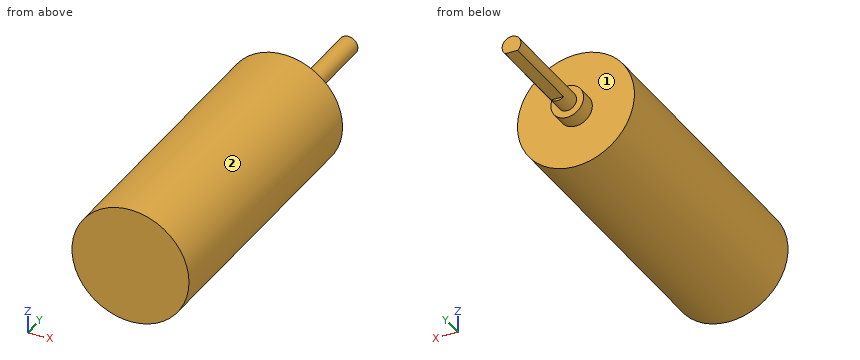
from build123d import *

# Parameters (mm, degrees)
SKETCH_1_R          = 12.5
EXTRUDE_1_DEPTH     = 62
SKETCH_2_R          = 3.5
EXTRUDE_2_DEPTH     = 3.5
SKETCH_3_R          = 2
EXTRUDE_3_DEPTH     = 22.5
CUT_EXTRUDE_1_DEPTH = 18.5


with BuildPart() as part:
    # 草图1 → 凸台-拉伸1 (new body)
    with BuildSketch(Plane(origin=(0, 0, 0), x_dir=(1, 0, 0), z_dir=(0, 1, 0))):
        Circle(SKETCH_1_R)
    extrude(amount=EXTRUDE_1_DEPTH)

    # 草图2 → 凸台-拉伸2 (add)
    with BuildSketch(Plane(origin=(0, 62, 0), x_dir=(1, 0, 0), z_dir=(0, 1, 0))):
        Circle(SKETCH_2_R)
    extrude(amount=EXTRUDE_2_DEPTH)

    # 草图3 → 凸台-拉伸3 (add)
    with BuildSketch(Plane(origin=(0, 65.5, 0), x_dir=(1, 0, 0), z_dir=(0, 1, 0))):
        Circle(SKETCH_3_R)
    extrude(amount=EXTRUDE_3_DEPTH)

    # 草图4 → 切除-拉伸1 (cut)
    with BuildSketch(Plane(origin=(0, 88, 0), x_dir=(1, 0, 0), z_dir=(0, 1, 0))):
        Polygon((-50.671161076, 1.5), (-1.322875656, 1.5), (1.322875656, 1.5), (50.671161076, 1.5), (50.671161076, 100.196570842), (-50.671161076, 100.196570842), align=None)
    extrude(amount=-CUT_EXTRUDE_1_DEPTH, mode=Mode.SUBTRACT)


solid = part.part
Input: part model. Units: mm. Frame: model coordinates. Face numbers are marked on the shaded views. A direction names the side the tool comes from. Give positions to 0.01 mm unless a question says otherwise; leave off trailing zeros. Loops run counter-clockwise (first coordinate to the right, second up) from the corner with the lowest first, then second, coordinate; pieces in that order, holes last. Notation, with made-up numbers: M 43,20.25 L 88,20.25 A18 ccw 88,47.25 Z; hole C 68,21.25 d8. An arc over 180 degrees is marked long. Use CSV: the item, a comma, the result in double quotes.
(1) Pin query (flat end, axial travel): P1, Ø4, axis at y = 77.5, z = -4.5, coming from the -X side; P2, Ø10, axis at x = -3.5, z = 5, coming from the +Y side; P3, Ø6, axis at y = 31.5, z = 6.5, coming from the +X side; P4, Ø3, axis at x = 0, y = 76, coming from the -Z side. Return the tip coordinate at first contact, or that it passes through.
Outcome:
P1,"passes through"
P2,"stops at y = 88"
P3,"stops at x = 12"
P4,"stops at z = -1.5"
(2) Set-up query: the marked faces 1 and 2. Return all of +Z, -Z, +X, -X, +Y, -Y with unobstructed straight access to the full face (end or side cutting, diameter ignored); none if empty.
Outcome:
face 1,"+Y"
face 2,"+Y, -Y"
(3) Section D-D, the plane y = 45.5. Return loops of the section in (x, z), plus the area to 3 significant figures.
Outcome:
outline,"C 0,0 d25"
area,"491 mm²"
(4) Section C-C, the plane y = 63.5. Return loops of the section in (x, z), plus the area to 3 significant figures.
Outcome:
outline,"C 0,0 d7"
area,"38.5 mm²"
(5) Section B-B, the plane z = 0. Return loops of the section in (x, y), plus the area to 3 significant figures.
Outcome:
outline,"M -12.5,0 L 12.5,0 L 12.5,62 L 3.5,62 L 3.5,65.5 L 2,65.5 L 2,88 L -2,88 L -2,65.5 L -3.5,65.5 L -3.5,62 L -12.5,62 Z"
area,"1,660 mm²"
(6) Section A-A, the plane x = 0. Return loops of the section in (y, z).
Outcome:
outline,"M 0,-12.5 L 62,-12.5 L 62,-3.5 L 65.5,-3.5 L 65.5,-2 L 69.5,-2 L 69.5,-1.5 L 88,-1.5 L 88,2 L 65.5,2 L 65.5,3.5 L 62,3.5 L 62,12.5 L 0,12.5 Z"
(7) Material intervals for L1, parallel to Y at x = -7.5, z = 8; L2, parallel to Z at x = 3.5, y = 42.5; L3, parallel to X at y = 29.5, z = 8.75, sorted ascending. Write a range as [from, to].
Outcome:
L1,"y = [0, 62]"
L2,"z = [-12, 12]"
L3,"x = [-8.93, 8.93]"
